The drawing under review shows one solid part. Ordinate dimensions are in mm from its lowest x, y, z. Give positions to 0.01 mm unless a question says otherwise; leave off trailing zeros. Loops run counter-clockwise (first coordinate to the right, second up) from the corner with the lowest first, then second, coordinate; pieces in that order, holes last. Notation, with made-up numbers: M 14,75.25 L 31,75.25 A10 ccw 31,88.25 Z; hole C 32.5,5.25 d1. An arc over 180 degrees is marked long. Answer as CSV lines item,"result".
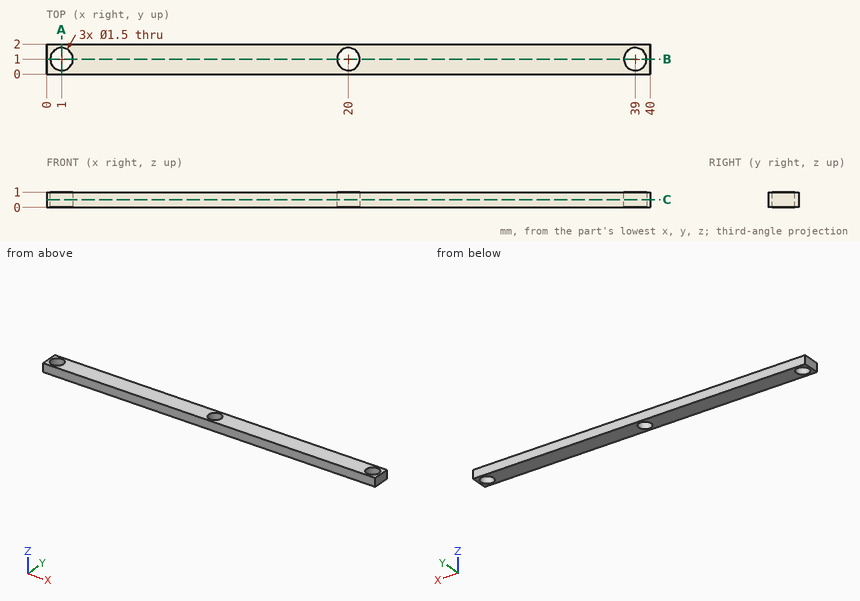
1. We need section B-B, the plane y = 1. Write out the cut boundary in (x, z).
Answer block:
outline,"M 0,0 L 0.25,0 L 0.25,1 L 0,1 Z; M 1.75,0 L 19.25,0 L 19.25,1 L 1.75,1 Z; M 20.75,0 L 38.25,0 L 38.25,1 L 20.75,1 Z; M 39.75,0 L 40,0 L 40,1 L 39.75,1 Z"
2. For P1, Ø1.2, axis at x = 39, y = 1, coming from the -Z side, flat-tipped, find the tip position at first contact; note if it passes through.
Answer block:
P1,"through"
3. We need section C-C, the plane z = 0.5. Write out the cut boundary in (x, y).
Answer block:
outline,"M 0,0 L 40,0 L 40,2 L 0,2 Z; hole C 1,1 d1.5; hole C 20,1 d1.5; hole C 39,1 d1.5"
4. To check wall thickness, follow L1, parallel to X at y = 0.95, z = 0.1; L2, parallel to Y at x = 39, z = 0.5; L3, parallel to X at y = 0.55, z = 0.8. State the ranges of each line that lie inside material, in increasing order. Write a range as [from, to].
Answer block:
L1,"[0, 0.25], [1.75, 19.25], [20.75, 38.25], [39.75, 40]"
L2,"[0, 0.25], [1.75, 2]"
L3,"[0, 0.4], [1.6, 19.4], [20.6, 38.4], [39.6, 40]"
5. We need section A-A, the plane x = 1. Write out the cut boundary in (y, z).
Answer block:
outline,"M 0,0 L 0.25,0 L 0.25,1 L 0,1 Z; M 1.75,0 L 2,0 L 2,1 L 1.75,1 Z"
